Can you work these out from the model? Positions are in its coordinate system, mm. Round coordinates to 2 decimals unless told otherwise and drop trailing zeros. Write each loop counter-clockwise with the first axis right and the second up, starting at its lowest first coordinate (ties: lowest second). Pieces come first, ordered by that corner, then holes. Notation, with made-up numbers: (-21.75, 15) -> (13.25, 15) arc R11 ccw to (13.25, 24) -> close; hole circle Ø10 at (76.25, 57). An arc over 180 degrees is marked (long way). Use CSV: the item, a comma, the result in double quotes.
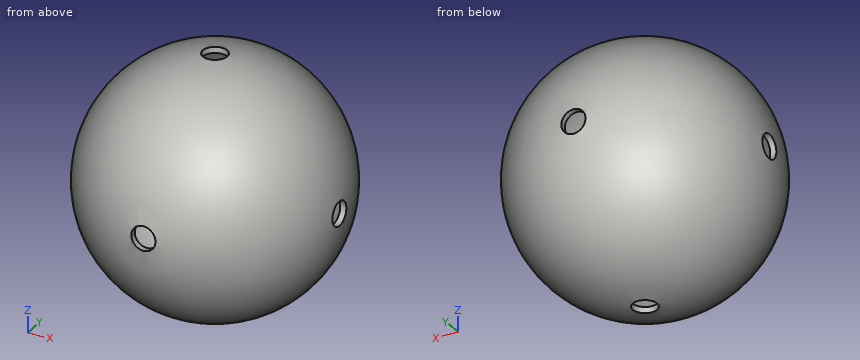
```python
from build123d import *

# Parameters (mm, degrees)
F2_T      = -0.75
F4_D      = 3
F4_DEPTH  = 15.501
F6_D      = 3
F8_D      = 3
F8_DEPTH  = 15.501
F10_D     = 3
F12_D     = 3
F12_DEPTH = 15.501
F14_D     = 3


# Not quite as in the source:
# - a feature names something its author has since deleted; it is built from what else it names


with BuildPart() as f1:
    # F0 (on Top) → F1 (revolve)
    with BuildSketch(Plane.XY):
        with BuildLine():
            ThreePointArc((15.5, 0), (0, 15.5), (-15.5, 0))
            Line((-15.5, 0), (15.5, 0))
        make_face()
    revolve(axis=Axis((0.5901393228, 0, 0), (1, 0, 0)))

    # F2 (hollow: no face is removed)
    offset(amount=F2_T, mode=Mode.SUBTRACT)

    # F4 (through all, one way)
    with BuildSketch(Plane.XY):
        with Locations((0, 0)):
            Circle(F4_D / 2)
    extrude(amount=-F4_DEPTH, mode=Mode.SUBTRACT)

    # F6 (through all)
    with Locations(Plane(origin=(0, 0, 0), x_dir=(1, 0, 0), z_dir=(0, 0, -1))):
        with Locations((0, 0)):
            Hole(F6_D / 2)

    # F8 (through all, one way)
    with BuildSketch(Plane.YZ):
        with Locations((0, 0)):
            Circle(F8_D / 2)
    extrude(amount=-F8_DEPTH, mode=Mode.SUBTRACT)

    # F10 (through all)
    with Locations(Plane(origin=(0, 0, 0), x_dir=(0, 1, 0), z_dir=(-1, 0, 0))):
        with Locations((0, 0)):
            Hole(F10_D / 2)

    # F12 (through all, one way)
    with BuildSketch(Plane.XZ):
        with Locations((0, 0)):
            Circle(F12_D / 2)
    extrude(amount=-F12_DEPTH, mode=Mode.SUBTRACT)

    # F14 (through all)
    with Locations(Plane(origin=(0, 0, 0), x_dir=(1, 0, 0), z_dir=(0, 1, 0))):
        with Locations((0, 0)):
            Hole(F14_D / 2)


solid = f1.part
```
Q1. Will these pins go through, and if not, where does the flat tip stop? P1, Ø3.5, axis at y = 0, z = 0, coming from the +X side; P2, Ø8, axis at x = 2.5, y = -10.5, coming from the -Z side; P3, Ø5, axis at y = 6, z = 1.5, coming from the +X side; P4, Ø4, axis at x = 9.5, y = 1, coming from the -Z side.
Resolved:
P1,"stops at x = 15.43"
P2,"stops at z = -13.93"
P3,"stops at x = 15.06"
P4,"stops at z = -13.54"
Q2. Suppose I cut it at D-D (z = -8). Write out the boundary of the cut face in (x, y).
Resolved:
outline,"circle Ø26.55 at (0, 0); hole circle Ø24.78 at (0, 0)"
Q3. Suppose I cut it at C-C (x = 13). Write out the boundary of the cut face in (y, z).
Resolved:
outline,"circle Ø16.88 at (0, 0); hole circle Ø13.94 at (0, 0)"
Q4. Suppose I cut it at A-A (y = 0). Write out the boundary of the cut face in (x, z), and give its area (3 significant figures).
Resolved:
outline,"(-15.43, -1.5) arc R15.5 ccw to (-1.5, -15.43) -> (-1.5, -14.67) arc R14.75 cw to (-14.67, -1.5) -> close; (-15.43, 1.5) -> (-14.67, 1.5) arc R14.75 cw to (-1.5, 14.67) -> (-1.5, 15.43) arc R15.5 ccw to start; (1.5, -15.43) arc R15.5 ccw to (15.43, -1.5) -> (14.67, -1.5) arc R14.75 cw to (1.5, -14.67) -> close; (1.5, 14.67) arc R14.75 cw to (14.67, 1.5) -> (15.43, 1.5) arc R15.5 ccw to (1.5, 15.43) -> close"
area,"62.3 mm^2"
Q5. Please list where these lines run through material, in increasing order: probe 1 along Y at (x, z) = (8, -0.5); probe 2 along Y at (x, z) = (0, 7.5); probe 3 along Z at (x, y) = (-5, -4).
Resolved:
probe 1,"y = -13.27 to -12.38, 12.38 to 13.27"
probe 2,"y = -13.56 to -12.7, 12.7 to 13.56"
probe 3,"z = -14.12 to -13.29, 13.29 to 14.12"
